from build123d import *

# Parameters (mm, degrees)
EXTRUDE_1_DEPTH       = 2
EXTRUDE_START         = 2.4
SKETCH_2_R            = 10
EXTRUDE_2_DEPTH       = 2.4
HOLE_WIZARD_2_0_2_1_D = 2
FILLET_1_R            = 20


with BuildPart() as part:
    # 草图1 → 凸台-拉伸1 (new body)
    with BuildSketch(Plane.XZ.offset(-2.4)):
        with BuildLine():
            Line((36.835257999, -98.834021309), (9.659258263, 2.588190451))
            ThreePointArc((9.659258263, 2.588190451), (0, 10), (-9.659258263, 2.588190451))
            Line((-9.659258263, 2.588190451), (-36.835257999, -98.834021309))
            ThreePointArc((-36.835257999, -98.834021309), (0, -105.475115549), (36.835257999, -98.834021309))
        make_face()
    extrude(amount=-EXTRUDE_1_DEPTH)

    # 草图2 → 凸台-拉伸2 (add)
    with BuildSketch(Plane.XZ.offset(-2.4).offset(EXTRUDE_START)):
        with Locations(Location((0, 0, 0), (0, 0, 270))):
            Circle(SKETCH_2_R)
    extrude(amount=-EXTRUDE_2_DEPTH)

    # Ø2.0 (2) 直径孔1 (through all)
    with Locations(Plane(origin=(0, 0, 0), x_dir=(-1, 0, 0), z_dir=(0, -1, 0))):
        with Locations((-6.958391143, -0.762097571), (-0.762097571, 6.958391143), (0.762097571, -6.958391143), (6.958391143, 0.762097571)):
            Hole(HOLE_WIZARD_2_0_2_1_D / 2)

    # 圆角1
    fillet_1_edges = [part.edges().sort_by_distance(p)[0] for p in [
        (-36.835257999, 3.4, -98.834021309),
        (36.835257999, 3.4, -98.834021309),
    ]]
    fillet(fillet_1_edges, radius=FILLET_1_R)


solid = part.part
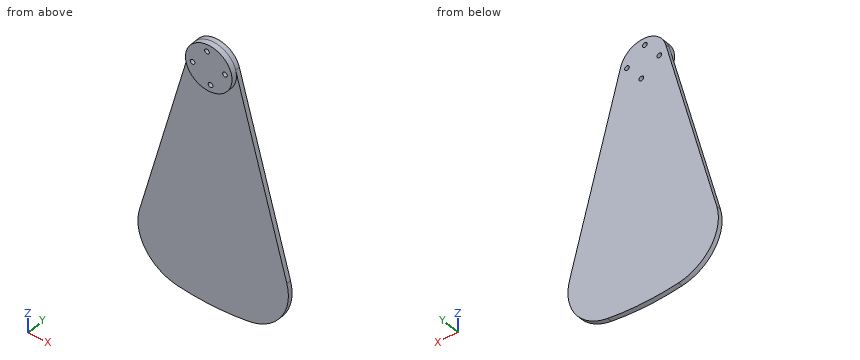
The listing builds one solid part. Answer for the finished solid, in the listing's coordinates (mm). Round coordinates to 2 decimals unless told otherwise and drop trailing zeros. Order: outer loops, then holes, each group sorted by start corner. A loop starts at its lowest first (then second) coordinate and runs counter-clockwise, first axis right, second up. Notation, with made-up numbers: (-37, 2.5) -> (-25, 2.5) arc R13 cw to (-25, 16.5) -> close; hole circle Ø10 at (88, -36). An arc over 180 degrees is marked (long way). Put each result on its own line as item: value.
Q1. Section A-A, the plane y = 3.6 is taken. Write down the section's boundary in (x, z), and give its area (3 significant figures).
Results list:
outline: (-31.63, -79.41) arc R20 ccw to (-15.19, -104.38) arc R105.48 ccw to (15.19, -104.38) arc R20 ccw to (31.63, -79.41) -> (9.66, 2.59) arc R10 ccw to (-9.66, 2.59) -> close; hole circle Ø2 at (-6.96, -0.76); hole circle Ø2 at (-0.76, 6.96); hole circle Ø2 at (0.76, -6.96); hole circle Ø2 at (6.96, 0.76)
area: 4,950 mm^2
Q2. Section B-B, the plane x = -14 is taken. Write down the section's boundary in (y, z), and give its area (3 significant figures).
Results list:
outline: (2.4, -104.54) -> (4.4, -104.54) -> (4.4, -13.61) -> (2.4, -13.61) -> close
area: 182 mm^2
Q3. Consider line 1 along Y through (x, z) = (10, -63.5); line 2 along X through (y, z) = (3.9, -10.5); line 3 along Z through (x, y) = (-1, 2.1). Determine where each line is inside the solid, lowest interval first.
Results list:
line 1: 2.4 to 4.4
line 2: -13.17 to 13.17
line 3: -9.95 to 5.99, 7.93 to 9.95
Q4. Each of these flat-tipped pins is pushed along its axis until it touches: P1, Ø2, axis at x = -25, y = 0.5, coming from the -Z side; P2, Ø10, axis at x = -7, z = -59, coming from the -Y side; P3, Ø2, axis at y = 2.5, z = -77, coming from the +X side. Where does it stop, or does it pass through?
Results list:
P1: through
P2: y = 2.4
P3: x = 31.25
Q5. Section C-C, the plane z = -62.5 is taken. Write down the section's boundary in (x, y).
Results list:
outline: (-27.1, 2.4) -> (27.1, 2.4) -> (27.1, 4.4) -> (-27.1, 4.4) -> close
